The listing builds one solid part. Answer for the finished solid, in the listing's coordinates (mm). A direction names the side the tool comes from. Round coordinates to 2 decimals unless told otherwise and drop trailing zeros. Write each loop counter-clockwise with the first axis right and the second up, starting at its lowest first coordinate (ties: lowest second). Pieces come first, ordered by that corner, then holes.
from build123d import *

# Parameters (mm, degrees)
SKETCH1_W           = 150
SKETCH1_H           = 150
BOSS_EXTRUDE1_DEPTH = 10
SKETCH3_W           = 12
SKETCH3_H           = 12
CUT_EXTRUDE2_DEPTH  = 107.536378763
CUT_EXTRUDE1_DEPTH  = 107.536378763
CIRPATTERN1_COUNT   = 4


with BuildPart() as part:
    # Sketch1 → Boss-Extrude1 (new body)
    with BuildSketch(Plane(origin=(0, 0, 0), x_dir=(1, 0, 0), z_dir=(0, 1, 0))):
        Rectangle(SKETCH1_W, SKETCH1_H)
    extrude(amount=BOSS_EXTRUDE1_DEPTH)

    # Sketch3 → Cut-Extrude2 (cut, through all)
    with BuildSketch(Plane(origin=(0, 10, 0), x_dir=(1, 0, 0), z_dir=(0, 1, 0))):
        Rectangle(SKETCH3_W, SKETCH3_H)
    extrude(amount=-CUT_EXTRUDE2_DEPTH, mode=Mode.SUBTRACT)

    # Sketch2 → Cut-Extrude1 (cut, through all)
    with BuildSketch(Plane(origin=(0, 10, 0), x_dir=(1, 0, 0), z_dir=(0, 1, 0))):
        with BuildLine():
            Line((20, 6), (55, 6))
            ThreePointArc((55, 6), (61, 0), (55, -6))
            Line((55, -6), (20, -6))
            ThreePointArc((20, -6), (14, 0), (20, 6))
        make_face()
    cut_extrude1 = extrude(amount=-CUT_EXTRUDE1_DEPTH, mode=Mode.SUBTRACT)

    # CirPattern1: Cut-Extrude1 ×4 about axis
    cirpattern1_axis = Axis((0, 0, 0), (0, 1, 0))
    for i in range(1, CIRPATTERN1_COUNT):
        add(cut_extrude1.rotate(cirpattern1_axis, i * 360 / CIRPATTERN1_COUNT), mode=Mode.SUBTRACT)


solid = part.part
1. Section D-D on y = 5 is taken. Determine the outline of the cut face in (x, z).
Geometry says:
outline: (-75, -75) - (75, -75) - (75, 75) - (-75, 75) - close; hole (-55, -6) - (-20, -6) arc R6 ccw to (-20, 6) - (-55, 6) arc R6 ccw to start; hole (-6, -55) arc R6 ccw to (6, -55) - (6, -20) arc R6 ccw to (-6, -20) - close; hole (-6, -6) - (6, -6) - (6, 6) - (-6, 6) - close; hole (-6, 20) arc R6 ccw to (6, 20) - (6, 55) arc R6 ccw to (-6, 55) - close; hole (20, -6) - (55, -6) arc R6 ccw to (55, 6) - (20, 6) arc R6 ccw to start
2. Section A-A on z = -48.5 is taken. Determine the outline of the cut face in (x, y), plus the area to 3 significant figures.
Geometry says:
outline: (-75, 0) - (-6, 0) - (-6, 10) - (-75, 10) - close; (6, 0) - (75, 0) - (75, 10) - (6, 10) - close
area: 1,380 mm2
3. For a pull along Z with two mould halves and no side action, classify faces 3 (the face through (-6, 5, -37)), 4 (the face through (-1, 5, -75)), 5 (the face through (-75, 5, 1)) as released by +Z, released by -Z, zero draft, split by the parting line, or undercut.
Geometry says:
face 3: undercut
face 4: released by -Z
face 5: zero draft
4. Straight lines are drawn through the part: line 1 along X through (y, z) = (2.75, 0); line 2 along X through (y, z) = (4.5, -26). For each, find the intervals that lie inside material, in ascending order.
Geometry says:
line 1: x = -75 to -61, -14 to -6, 6 to 14, 61 to 75
line 2: x = -75 to -6, 6 to 75
5. Section C-C on x = 0 is taken. Determine the outline of the cut face in (y, z), plus the area to 3 significant figures.
Geometry says:
outline: (0, -75) - (10, -75) - (10, -61) - (0, -61) - close; (0, -14) - (10, -14) - (10, -6) - (0, -6) - close; (0, 6) - (10, 6) - (10, 14) - (0, 14) - close; (0, 61) - (10, 61) - (10, 75) - (0, 75) - close
area: 440 mm2
6. Section B-B on z = 0 is taken. Determine the outline of the cut face in (x, y).
Geometry says:
outline: (-75, 0) - (-61, 0) - (-61, 10) - (-75, 10) - close; (-14, 0) - (-6, 0) - (-6, 10) - (-14, 10) - close; (6, 0) - (14, 0) - (14, 10) - (6, 10) - close; (61, 0) - (75, 0) - (75, 10) - (61, 10) - close
7. A tool of negligible diameter and unlimited length cuts with its end or side. For faces 1 (the face through (-1, 5, 75)), 2 (the face through (0, 5, 61)), from which of +Z, -Z, +X, -X, +Y, -Y can it reach the whole face along a straight path? Write none if from no direction.
Geometry says:
face 1: +Z, +X, -X, +Y, -Y
face 2: +Y, -Y
